from build123d import *

# Parameters (mm, degrees)
F1_DEPTH = 25.4


with BuildPart() as f1:
    # F0 (on Front) → F1 (new body)
    with BuildSketch(Plane.XZ):
        with BuildLine():
            ThreePointArc((-41.1120045974, 60.4052241132), (-38.8054616332, 52.9144038037), (-31.6617116332, 49.6895991132))
            ThreePointArc((-31.6617116332, 49.6895991132), (-24.9265195424, 52.4794070224), (-22.1367116332, 59.2145991132))
            ThreePointArc((-22.1367116332, 59.2145991132), (-22.155406739, 59.8110823551), (-22.211418669, 60.4052241132))
            ThreePointArc((-22.211418669, 60.4052241132), (-31.6617116332, 68.7395991132), (-41.1120045974, 60.4052241132))
        make_face()
        with BuildLine():
            ThreePointArc((-28.4867116332, 59.2145991132), (-29.4166476029, 56.9695350829), (-31.6617116332, 56.0395991132))
            ThreePointArc((-31.6617116332, 56.0395991132), (-33.9067756635, 61.4596631434), (-28.4867116332, 59.2145991132))
        make_face(mode=Mode.SUBTRACT)
        with BuildLine():
            ThreePointArc((-22.1367116332, 59.2145991132), (-24.9265195424, 52.4794070224), (-31.6617116332, 49.6895991132))
            Line((-31.6617116332, 49.6895991132), (-31.6617116332, 24.2895991132))
            ThreePointArc((-31.6617116332, 24.2895991132), (-21.1613861174, 20.3208491132), (-15.9112233595, 10.3989741132))
            Line((-15.9112233595, 10.3989741132), (-22.211418669, 60.4052241132))
            ThreePointArc((-22.211418669, 60.4052241132), (-22.155406739, 59.8110823551), (-22.1367116332, 59.2145991132))
        make_face()
        with BuildLine():
            Line((-31.6617116332, 24.2895991132), (-31.6617116332, 49.6895991132))
            ThreePointArc((-31.6617116332, 49.6895991132), (-38.8054616332, 52.9144038037), (-41.1120045974, 60.4052241132))
            Line((-41.1120045974, 60.4052241132), (-47.4121999069, 10.3989741132))
            ThreePointArc((-47.4121999069, 10.3989741132), (-42.162037149, 20.3208491132), (-31.6617116332, 24.2895991132))
        make_face()
        with BuildLine():
            ThreePointArc((-15.9112233595, 10.3989741132), (-21.1613861174, 20.3208491132), (-31.6617116332, 24.2895991132))
            Line((-31.6617116332, 24.2895991132), (-31.6617116332, 11.5895991132))
            ThreePointArc((-31.6617116332, 11.5895991132), (-29.4166476029, 10.6596631434), (-28.4867116332, 8.4145991132))
            ThreePointArc((-28.4867116332, 8.4145991132), (-29.4166476029, 6.1695350829), (-31.6617116332, 5.2395991132))
            Line((-31.6617116332, 5.2395991132), (-31.6617116332, -7.4604008868))
            ThreePointArc((-31.6617116332, -7.4604008868), (-21.0124378904, -3.3586159851), (-15.8662860691, 6.8270991132))
            ThreePointArc((-15.8662860691, 6.8270991132), (-15.8066177226, 7.6198525591), (-15.7867116332, 8.4145991132))
            ThreePointArc((-15.7867116332, 8.4145991132), (-15.8178701428, 9.4087378498), (-15.9112233595, 10.3989741132))
        make_face()
        with BuildLine():
            Line((-31.6617116332, 11.5895991132), (-31.6617116332, 24.2895991132))
            ThreePointArc((-31.6617116332, 24.2895991132), (-42.162037149, 20.3208491132), (-47.4121999069, 10.3989741132))
            ThreePointArc((-47.4121999069, 10.3989741132), (-47.5354554487, 8.6143045999), (-47.4571371973, 6.8270991132))
            ThreePointArc((-47.4571371973, 6.8270991132), (-42.310985376, -3.3586159851), (-31.6617116332, -7.4604008868))
            Line((-31.6617116332, -7.4604008868), (-31.6617116332, 5.2395991132))
            ThreePointArc((-31.6617116332, 5.2395991132), (-34.8367116332, 8.4145991132), (-31.6617116332, 11.5895991132))
        make_face()
        with BuildLine():
            ThreePointArc((-31.6617116332, -7.4604008868), (-42.310985376, -3.3586159851), (-47.4571371973, 6.8270991132))
            Line((-47.4571371973, 6.8270991132), (-41.1389669716, -56.0379008868))
            ThreePointArc((-41.1389669716, -56.0379008868), (-38.7256406922, -48.6958366411), (-31.6617116332, -45.5604008868))
            Line((-31.6617116332, -45.5604008868), (-31.6617116332, -7.4604008868))
        make_face()
        with BuildLine():
            ThreePointArc((-15.8662860691, 6.8270991132), (-21.0124378904, -3.3586159851), (-31.6617116332, -7.4604008868))
            Line((-31.6617116332, -7.4604008868), (-31.6617116332, -45.5604008868))
            ThreePointArc((-31.6617116332, -45.5604008868), (-24.9265195424, -48.350208796), (-22.1367116332, -55.0854008868))
            Line((-22.1367116332, -55.0854008868), (4.8507883668, -55.0854008868))
            ThreePointArc((4.8507883668, -55.0854008868), (7.2767655853, -49.3733939821), (13.0717705097, -47.1529646832))
            Line((13.0717705097, -47.1529646832), (-12.6941116327, -46.232167176))
            ThreePointArc((-12.6941116327, -46.232167176), (-18.4005117359, -43.514041737), (-20.3205250409, -37.4920190744))
            Line((-20.3205250409, -37.4920190744), (-15.8662860691, 6.8270991132))
        make_face()
        with BuildLine():
            ThreePointArc((-31.6617116332, -45.5604008868), (-38.7256406922, -48.6958366411), (-41.1389669716, -56.0379008868))
            ThreePointArc((-41.1389669716, -56.0379008868), (-37.9240950148, -62.2623207959), (-31.3215330618, -64.6043243312))
            ThreePointArc((-31.3215330618, -64.6043243312), (-24.8073033476, -61.6992282246), (-22.1367116332, -55.0854008868))
            Line((-22.1367116332, -55.0854008868), (-28.4867116332, -55.0854008868))
            ThreePointArc((-28.4867116332, -55.0854008868), (-33.9067756635, -57.3304649171), (-31.6617116332, -51.9104008868))
            Line((-31.6617116332, -51.9104008868), (-31.6617116332, -45.5604008868))
        make_face()
        with BuildLine():
            ThreePointArc((-22.1367116332, -55.0854008868), (-24.8073033476, -61.6992282246), (-31.3215330618, -64.6043243312))
            Line((-31.3215330618, -64.6043243312), (13.0717705097, -63.0178370905))
            ThreePointArc((13.0717705097, -63.0178370905), (7.2767655853, -60.7974077915), (4.8507883668, -55.0854008868))
            Line((4.8507883668, -55.0854008868), (-22.1367116332, -55.0854008868))
        make_face()
        with BuildLine():
            ThreePointArc((4.8507883668, -55.0854008868), (7.2767655853, -60.7974077915), (13.0717705097, -63.0178370905))
            ThreePointArc((13.0717705097, -63.0178370905), (18.5002952715, -60.5969236683), (20.7257883668, -55.0854008868))
            ThreePointArc((20.7257883668, -55.0854008868), (18.5002952715, -49.5738781054), (13.0717705097, -47.1529646832))
            ThreePointArc((13.0717705097, -47.1529646832), (7.2767655853, -49.3733939821), (4.8507883668, -55.0854008868))
        make_face()
        with BuildLine():
            ThreePointArc((15.9632883668, -55.0854008868), (12.7882883668, -58.2604008868), (9.6132883668, -55.0854008868))
            ThreePointArc((9.6132883668, -55.0854008868), (12.7882883668, -51.9104008868), (15.9632883668, -55.0854008868))
        make_face(mode=Mode.SUBTRACT)
        with BuildLine():
            ThreePointArc((-22.1367116332, -55.0854008868), (-24.9265195424, -48.350208796), (-31.6617116332, -45.5604008868))
            Line((-31.6617116332, -45.5604008868), (-31.6617116332, -51.9104008868))
            ThreePointArc((-31.6617116332, -51.9104008868), (-29.4166476029, -52.8403368566), (-28.4867116332, -55.0854008868))
            Line((-28.4867116332, -55.0854008868), (-22.1367116332, -55.0854008868))
        make_face()
    extrude(amount=F1_DEPTH)


solid = f1.part
CAD build for the part. Positions are in the model's coordinates, mm. Round coordinates to 2 decimals unless told otherwise and drop trailing zeros. Loops run counter-clockwise (first coordinate to the right, second up) from the corner with the lowest first, then second, coordinate; pieces in that order, holes last.
(1) Cut at A-A (y = -12.25). State how many separate pieces and enclosed holes the cut face has, plus the area to 3 significant figures.
(2) Drop flat-ended pins along their axis: pin 1 (4 mm diameter, centred on x = -8.5, y = -21.5, fed in from +Z); pin 2 (2 mm diameter, centred on y = -17.5, z = -20.5, fed in from +X); pin 3 (1.5 mm diameter, centred on x = -37, y = -17, fed in from -Z). Give the stop position or say it passes through.
(3) Wall check: line 1 along Z through (x, y) = (-32, -21); line 2 along Z through (x, y) = (-30, -8.5); line 3 along X through (y, z) = (-8.5, -57.5). Give the ranges that are in metal, low to high.
(4) Cut at B-B (z = 43.5). Give the cut face in (x, y).
(5) Cut at C-C (x = 4). Give the cut face in (y, z), plus the area to 3 significant figures.
(6) Two-plate mould, pull along Z, no slides. Class faces 1 (the flat face through (-19.017, -12.522, 35.052)), 2 (the flat face through (-18.125, -12.522, -15.643)), 3 (the flat face through (-29, 0, -12)): +Z half, -Z half, draft (parallel to the pull), parting line (faces both ways), or undercut.
Findings below:
1. separate pieces: 1
1. enclosed holes: 4
1. area: 3,810 mm2
2. pin 1: stops at z = -46.31
2. pin 2: stops at x = -18.51
2. pin 3: stops at z = -63.43
3. line 1: z = -64.6 to -58.24, -51.93 to 5.26, 11.57 to 56.06, 62.37 to 68.73
3. line 2: z = -64.56 to -57.79, -52.38 to 5.71, 11.12 to 56.51, 61.92 to 68.59
3. line 3: x = -40.88 to -33.72, -29.6 to 10.73, 14.85 to 20.35
4. outline: (-43.24, -25.4) - (-20.08, -25.4) - (-20.08, 0) - (-43.24, 0) - close
5. outline: (-25.4, -63.34) - (0, -63.34) - (0, -46.83) - (-25.4, -46.83) - close
5. area: 419 mm2
6. face 1: +Z half
6. face 2: undercut
6. face 3: draft
